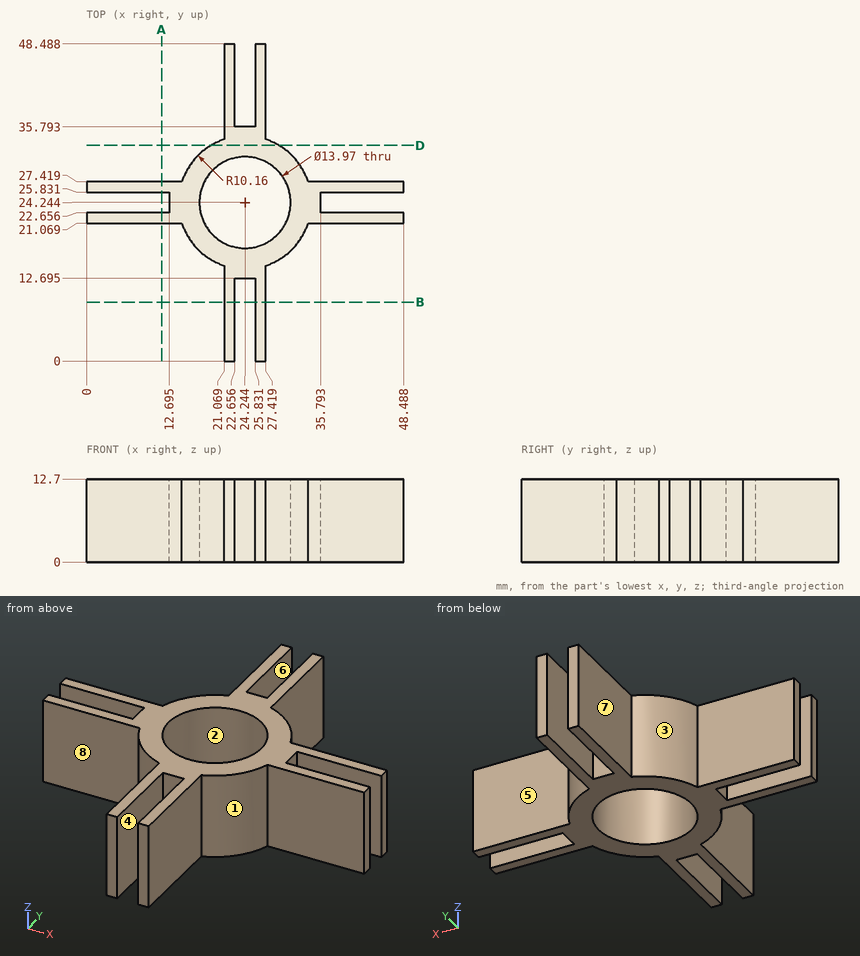
Part print with two shaded views. Sizes in mm from the minimum x, y, z corner. A direction names the side the tool comes from. Give positions to 0.01 mm unless a question says otherwise; leave off trailing zeros. Write each loop counter-clockwise with the first axis right and the second up, starting at its lowest first coordinate (ties: lowest second). Pieces come first, ordered by that corner, then holes.
1) Two-plate mould, pull along X, no slides. Class the marked faces 1, 2 and 3: released by +X, released by -X, zero draft, split by the parting line, or undercut.
Resolved:
face 1: released by +X
face 2: undercut
face 3: released by -X
2) Cut at A-A on x = 11.5. Write the cut outline in (y, z).
Resolved:
outline: (21.07, 0) - (22.66, 0) - (22.66, 12.7) - (21.07, 12.7) - close; (25.83, 0) - (27.42, 0) - (27.42, 12.7) - (25.83, 12.7) - close
3) Probe L1, parallel to Y at x = 24, z = 2 (1 decimal); L2, parallel to X at y = 43, z = 5.5. List the from-to ranges inside material, lowest first.
Resolved:
L1: y = 12.7 to 17.3, 31.2 to 35.8
L2: x = 21.07 to 22.66, 25.83 to 27.42
4) Pin check, flat tips, straight feed: pin 1 (6.5 mm diameter, centred on x = 43.5, z = 4, fed in from +Y); pin 2 (1.5 mm diameter, centred on x = 39.5, z = 8, fed in from -Y); pin 3 (6 mm diameter, centred on x = 13, z = 8.5, fed in from +Y). Stop position of each tip, or through.
Resolved:
pin 1: stops at y = 27.42
pin 2: stops at y = 21.07
pin 3: stops at y = 30.18
5) Which spindle directions (+Z, -Z, +X, -X, +Y, -Y) get a long thin tool onto all of the face, cutting with end or side? Do the marked faces 4, 5, 6, 7 and 8. Say none if no direction does.
Resolved:
face 4: +Z, -Z, -Y
face 5: +Z, -Z, +X, +Y
face 6: +Z, -Z, +Y
face 7: +Z, -Z, -X, +Y
face 8: +Z, -Z, -X, -Y
6) Cut at D-D on y = 33. Write the cut outline in (x, z).
Resolved:
outline: (19.09, 0) - (29.4, 0) - (29.4, 12.7) - (19.09, 12.7) - close
